Part model, mm, in its own coordinate system. A direction names the side the tool comes from. Give positions to 0.01 mm unless a question says otherwise; leave off trailing zeros. Order: outer loops, then holes, each group sorted by start corner. A loop starts at its lowest first (then second) coordinate and runs counter-clockwise, first axis right, second up. Notation, with made-up numbers: (-2.75, 40) - (44.25, 40) arc R11 ccw to (44.25, 46) - close; hole circle Ø4 at (41.5, -30.5). An arc over 180 degrees is marked (long way). Use one line per item in the form item = value. Start each with the question number.
1. Pin check, flat tips, straight feed: P1, Ø3.5, axis at x = 3, z = 9, coming from the -Y side; P2, Ø1, axis at y = 2, z = 41.5, coming from the +X side. Stop position of each tip, or through.
2. Pull direction Z, two halves, no side cores. Call faces 1 (the face through (-10.24, 1.48, 56.45)), 2 (the face through (61.976, 1, -26)), 3 (the face through (41.406, 1.521, 29.568)): +Z half, -Z half, draft (parallel to the pull), parting line (faces both ways), or undercut.
3. Band-saw the part on C-C, the plane x = 49.5. List the corners of the cut face in (y, z), plus the area to 3 significant figures.
4. Band-saw the part on D-D, the plane y = 1.6. State how many separate pieces and enclosed holes the cut face has, plus the area to 3 significant figures.
5. Tool access for faces 4 (the face through (49.73, 1.48, 17.72)), 5 (the face through (13.631, 1.479, -52.997)): list every direction of +Z, -Z, +X, -X, +Y, -Y with a clear straight run to the whole face (end or side of a thin tool).
6. Drill centre lines: line 1 (X direction, y = 1.25, z = 28.5); line 2 (X direction, y = 0.65, z = -32); line 3 (Z direction, x = -25.5, y = 0.6). Where is each one in solid material? Low to high.
7. Band-saw the part on A-A, the plane x = 9. List the corners of the cut face in (y, z), plus the area to 3 significant figures.
8. Band-saw the part on B-B, the plane z = 15. List the corners of the cut face in (x, y).
from build123d import *
from build123d.topology import SkipClean

# Parameters (mm, degrees)
SKETCH_1_R               = 1.55
SKETCH_1_R_2             = 4
EXTRUDE_1_DEPTH          = 3
EXTRUDE_START            = -3
SKETCH_2_R               = 2.1
EXTRUDE_3_DEPTH          = 3
FILLET_1_R               = 4
FILLET_2_R               = 314
FILLET_3_R               = 314
FILLET_4_R               = 4
CUT_EXTRUDE_2_DEPTH      = 3
EXTRUDE_4_DEPTH          = 3
CUT_EXTRUDE_START        = -10
SKETCH_5_R               = 22.5
CUT_EXTRUDE_3_DEPTH      = 10
SKETCH_6_R               = 13.5
EXTRUDE_5_DEPTH          = 3
EXTRUDE_6_DEPTH          = 3
CUT_EXTRUDE_5_DEPTH      = 98.662684788
CUT_EXTRUDE_5_DEPTH_BACK = 3
SKETCH_9_R               = 1.55
CUT_EXTRUDE_7_DEPTH      = 10
SKETCH_10_W              = 64.519287894
SKETCH_10_H              = 7.041569679
EXTRUDE_7_DEPTH          = 3
SKETCH_11_R              = 1.55
CUT_EXTRUDE_8_DEPTH      = 10


with BuildPart() as part:
    # 草图1 → 凸台-拉伸1 (new body)
    with BuildSketch(Plane(origin=(0, 0, 0), x_dir=(1, 0, 0), z_dir=(0, 1, 0))):
        with BuildLine():
            Line((-27.819418646, 37.14796354), (-55, 11))
            Line((-55, 11), (-55, -11))
            Line((-55, -11), (-27.819418646, -37.14796354))
            ThreePointArc((-27.819418646, -37.14796354), (-23.984664844, -39.630488814), (-19.5, -40.5))
            Line((-19.5, -40.5), (-17.421399483, -40.31860482))
            Line((-17.421399483, -40.31860482), (45.042813224, -34.867481809))
            ThreePointArc((45.042813224, -34.867481809), (58.724014778, -30.74585061), (69.617928959, -21.5))
            Line((69.617928959, -21.5), (19, -21.5))
            ThreePointArc((19, -21.5), (15.464466094, -20.035533906), (14, -16.5))
            Line((14, -16.5), (14, -12.539936204))
            ThreePointArc((14, -12.539936204), (5.5, 0), (14, 12.539936204))
            Line((14, 12.539936204), (14, 16.5))
            ThreePointArc((14, 16.5), (15.464466094, 20.035533906), (19, 21.5))
            Line((19, 21.5), (69.617928959, 21.5))
            ThreePointArc((69.617928959, 21.5), (58.724014778, 30.74585061), (45.042813224, 34.867481809))
            Line((45.042813224, 34.867481809), (-17.421399483, 40.31860482))
            Line((-17.421399483, 40.31860482), (-19.5, 40.5))
            ThreePointArc((-19.5, 40.5), (-23.984664844, 39.630488814), (-27.819418646, 37.14796354))
        make_face()
        with Locations(Location((-29, -28.5, 0), (0, 0, 270))):
            Circle(SKETCH_1_R, mode=Mode.SUBTRACT)
        with Locations(Location((-19.5, -36.5, 0), (0, 0, 270))):
            Circle(SKETCH_1_R, mode=Mode.SUBTRACT)
        with Locations(Location((-19.5, -28.5, 0), (0, 0, 270))):
            Circle(SKETCH_1_R_2, mode=Mode.SUBTRACT)
        with Locations(Location((-10, -28.5, 0), (0, 0, 270))):
            Circle(SKETCH_1_R, mode=Mode.SUBTRACT)
        with Locations(Location((-19.5, -20.5, 0), (0, 0, 270))):
            Circle(SKETCH_1_R, mode=Mode.SUBTRACT)
        with Locations(Location((-46.5, 0, 0), (0, 0, 270))):
            Circle(SKETCH_1_R, mode=Mode.SUBTRACT)
        with Locations(Location((-27.5, 0, 0), (0, 0, 270))):
            Circle(SKETCH_1_R, mode=Mode.SUBTRACT)
        with Locations(Location((0, 0, 0), (0, 0, 270))):
            Circle(SKETCH_1_R, mode=Mode.SUBTRACT)
        with Locations(Location((-29, 28.5, 0), (0, 0, 270))):
            Circle(SKETCH_1_R, mode=Mode.SUBTRACT)
        with Locations(Location((-19.5, 20.5, 0), (0, 0, 270))):
            Circle(SKETCH_1_R, mode=Mode.SUBTRACT)
        with Locations(Location((-19.5, 28.5, 0), (0, 0, 270))):
            Circle(SKETCH_1_R_2, mode=Mode.SUBTRACT)
        with Locations(Location((-10, 28.5, 0), (0, 0, 270))):
            Circle(SKETCH_1_R, mode=Mode.SUBTRACT)
        with Locations(Location((-19.5, 36.5, 0), (0, 0, 270))):
            Circle(SKETCH_1_R, mode=Mode.SUBTRACT)
    extrude(amount=EXTRUDE_1_DEPTH)

    # 草图2 → 凸台-拉伸3 (add)
    with BuildSketch(Plane(origin=(0, 3, 0), x_dir=(1, 0, 0), z_dir=(0, 1, 0)).offset(EXTRUDE_START)):
        with BuildLine():
            Line((-7, 60), (-28.363974347, 36.588878709))
            ThreePointArc((-28.363974347, 36.588878709), (-26.665503977, 38.125775437), (-24.705947863, 39.311942788))
            Line((-24.705947863, 39.311942788), (-19.656872495, 39.177623495))
            Line((-19.656872495, 39.177623495), (-17.421399483, 40.31860482))
            Line((-17.421399483, 40.31860482), (17, 37.314720281))
            Line((17, 37.314720281), (17, 50))
            Line((17, 50), (17, 60))
            Line((17, 60), (-7, 60))
        make_face()
        with Locations(Location((13, 55, 0), (0, 0, 270))):
            Circle(SKETCH_2_R, mode=Mode.SUBTRACT)
        with Locations(Location((-3, 55, 0), (0, 0, 270))):
            Circle(SKETCH_2_R, mode=Mode.SUBTRACT)
    extrude_3 = extrude(amount=EXTRUDE_3_DEPTH)

    # 圆角1
    fillet_1_edges = [part.edges().sort_by_distance(p)[0] for p in [
        (17, 1.5, -37.314720281),
    ]]
    fillet(fillet_1_edges, radius=FILLET_1_R)

    # 圆角2
    # the kernel refuses this fillet: 314 mm, written as the material it adds along each edge
    with BuildSketch(Plane(origin=(-28.100791786, 0, -36.877280051), x_dir=(0.6740732257670936, 0, -0.7386645289330906), z_dir=(0, 1, 0))) as fillet_2_piece_1:
        with BuildLine():
            CenterArc((FILLET_2_R * 0.032536346624, FILLET_2_R), FILLET_2_R, 266.272924122, 3.727075878)
            Line((-FILLET_2_R * 0.0324675326171, FILLET_2_R * 0.0021149887469), (0, 0))
            Line((0, 0), (FILLET_2_R * 0.032536346624, 0))
        make_face()
    extrude(amount=3)

    # 镜向2: 凸台-拉伸3 across plane
    add(extrude_3.mirror(Plane.XY))

    # 圆角3
    # the kernel refuses this fillet: 314 mm, written as the material it adds along each edge
    with BuildSketch(Plane(origin=(-28.100791786, 0, 36.877280051), x_dir=(-0.7206636283184775, 0, -0.6932848871992288), z_dir=(0, 1, 0))) as fillet_3_piece_1:
        with BuildLine():
            CenterArc((FILLET_3_R * 0.0325363466241, FILLET_3_R), FILLET_3_R, 266.272924122, 3.727075878)
            Line((-FILLET_3_R * 0.0324675326171, FILLET_3_R * 0.0021149887469), (0, 0))
            Line((0, 0), (FILLET_3_R * 0.032536346624, 0))
        make_face()
    extrude(amount=3)

    # 圆角4
    fillet_4_edges = [part.edges().sort_by_distance(p)[0] for p in [
        (17, 1.5, 37.314720281),
    ]]
    fillet(fillet_4_edges, radius=FILLET_4_R)

    # 草图3 → 切除-拉伸2 (cut)
    with BuildSketch(Plane.XZ):
        with BuildLine():
            ThreePointArc((-8.686732059, 48.231275591), (-35.637539634, 44.178960889), (-38.911435654, 17.122558906))
            ThreePointArc((-38.911435654, 17.122558906), (-32.411561674, 15.426493388), (-30.715496156, 21.926367368))
            ThreePointArc((-30.715496156, 21.926367368), (-28.823911789, 37.55895518), (-13.252334078, 39.900292563))
            ThreePointArc((-13.252334078, 39.900292563), (-6.804041555, 41.782983067), (-8.686732059, 48.231275591))
        make_face()
    cut_extrude_2 = extrude(amount=-CUT_EXTRUDE_2_DEPTH, mode=Mode.SUBTRACT)

    # 草图4 → 凸台-拉伸4 (add)
    with SkipClean():  # the faces are left unmerged after this step: merging them gives an invalid solid
        with BuildSketch(Plane.XZ):
            with BuildLine():
                Line((-43.624805935, 21.943038922), (-41.535713139, 23.952764967))
                ThreePointArc((-41.535713139, 23.952764967), (-35.617955509, 44.199092655), (-15.534428758, 50.647781937))
                Line((-15.534428758, 50.647781937), (-13.580394358, 52.78905657))
                ThreePointArc((-13.580394358, 52.78905657), (-37.408839455, 45.943436284), (-43.624805935, 21.943038922))
            make_face()
            with BuildLine():
                ThreePointArc((-25.118289886, 40.223259732), (-28.812596517, 37.570586867), (-31.367097826, 33.807729194))
                ThreePointArc((-31.367097826, 33.807729194), (-28.219819959, 36.993214998), (-25.118289886, 40.223259732))
            make_face()
        extrude_4 = extrude(amount=-EXTRUDE_4_DEPTH)

    # 镜向9: 切除-拉伸2, 凸台-拉伸4 across plane
    with SkipClean():  # the faces are left unmerged after this step: merging them gives an invalid solid
        add(cut_extrude_2.mirror(Plane.XY), mode=Mode.SUBTRACT)
        add(extrude_4.mirror(Plane.XY))

    # 草图5 → 切除-拉伸3 (cut)
    with SkipClean():  # the faces are left unmerged after this step: merging them gives an invalid solid
        with BuildSketch(Plane(origin=(0, 3, 0), x_dir=(1, 0, 0), z_dir=(0, 1, 0)).offset(CUT_EXTRUDE_START)):
            with Locations(Location((-19.5, 28.5, 0), (0, 0, 270))):
                Circle(SKETCH_5_R)
            with Locations(Location((-19.5, -28.5, 0), (0, 0, 90))):
                Circle(SKETCH_5_R)
        extrude(amount=CUT_EXTRUDE_3_DEPTH, mode=Mode.SUBTRACT)

    # 草图6 → 凸台-拉伸5 (add)
    with SkipClean():  # the faces are left unmerged after this step: merging them gives an invalid solid
        with BuildSketch(Plane(origin=(0, 3, 0), x_dir=(1, 0, 0), z_dir=(0, 1, 0)).offset(EXTRUDE_START)):
            with BuildLine():
                ThreePointArc((7.831521739, -7.583870604), (77, 0), (7.831521739, 7.583870604))
                ThreePointArc((7.831521739, 7.583870604), (5.5, 0), (7.831521739, -7.583870604))
            make_face()
            with Locations(Location((42, 0, 0), (0, 0, 270))):
                Circle(SKETCH_6_R, mode=Mode.SUBTRACT)
        extrude(amount=EXTRUDE_5_DEPTH)

    # 草图7 → 凸台-拉伸6 (add)
    with SkipClean():  # the faces are left unmerged after this step: merging them gives an invalid solid
        with BuildSketch(Plane(origin=(0, 3, 0), x_dir=(1, 0, 0), z_dir=(0, 1, 0)).offset(EXTRUDE_START)):
            with BuildLine():
                Line((17, 60), (61.975534644, 28.739833258))
                ThreePointArc((61.975534644, 28.739833258), (53.910000161, 32.911273086), (45.042813224, 34.867481809))
                Line((45.042813224, 34.867481809), (20.652249917, 36.995995963))
                ThreePointArc((20.652249917, 36.995995963), (18.051186651, 38.278167206), (17, 40.980851027))
                Line((17, 40.980851027), (17, 60))
            make_face()
            with BuildLine():
                Line((17, -60), (61.975557807, -28.739817159))
                ThreePointArc((61.975557807, -28.739817159), (53.910013423, -32.911268287), (45.042813224, -34.867481809))
                Line((45.042813224, -34.867481809), (20.652249917, -36.995995963))
                ThreePointArc((20.652249917, -36.995995963), (18.051186651, -38.278167206), (17, -40.980851027))
                Line((17, -40.980851027), (17, -60))
            make_face()
        extrude(amount=EXTRUDE_6_DEPTH)

    # 草图8 → 切除-拉伸5 (cut, two sides: drawn at the far end of the back side and taken through both)
    with SkipClean():  # the faces are left unmerged after this step: merging them gives an invalid solid
        with BuildSketch(Plane(origin=(0, 3, 0), x_dir=(1, 0, 0), z_dir=(0, 1, 0)).offset(-CUT_EXTRUDE_5_DEPTH_BACK)):
            with BuildLine():
                Line((61.975534644, 28.739833258), (61.975534644, 22.739833258))
                Line((61.975534644, 22.739833258), (35.963826017, 12.075371781))
                Line((35.963826017, 12.075371781), (35.963826017, -12.075371781))
                Line((35.963826017, -12.075371781), (61.975534644, -22.739833258))
                Line((61.975534644, -22.739833258), (61.975534644, -28.739833258))
                ThreePointArc((61.975534644, -28.739833258), (77, 1.4104e-05), (61.975534644, 28.739833258))
            make_face()
        extrude(amount=CUT_EXTRUDE_5_DEPTH + CUT_EXTRUDE_5_DEPTH_BACK, mode=Mode.SUBTRACT)

    # 草图9 → 切除-拉伸7 (cut)
    with SkipClean():  # the faces are left unmerged after this step: merging them gives an invalid solid
        with BuildSketch(Plane(origin=(0, 3, 0), x_dir=(1, 0, 0), z_dir=(0, 1, 0))):
            with Locations(Location((-53, -9, 0), (0, 0, 270))):
                Circle(SKETCH_9_R)
            with Locations(Location((-53, 9, 0), (0, 0, 270))):
                Circle(SKETCH_9_R)
            with Locations(Location((3, 9, 0), (0, 0, 270))):
                Circle(SKETCH_9_R)
            with Locations(Location((3, -9, 0), (0, 0, 270))):
                Circle(SKETCH_9_R)
        extrude(amount=-CUT_EXTRUDE_7_DEPTH, mode=Mode.SUBTRACT)

    # 草图10 → 凸台-拉伸7 (add)
    with SkipClean():  # the faces are left unmerged after this step: merging them gives an invalid solid
        with BuildSketch(Plane(origin=(0, 3, 0), x_dir=(1, 0, 0), z_dir=(0, 1, 0))):
            with Locations((-17.723905758, 0.445902683)):
                Rectangle(SKETCH_10_W, SKETCH_10_H)
        extrude(amount=-EXTRUDE_7_DEPTH)

    # 草图11 → 切除-拉伸8 (cut)
    with SkipClean():  # the faces are left unmerged after this step: merging them gives an invalid solid
        with BuildSketch(Plane(origin=(0, 3, 0), x_dir=(1, 0, 0), z_dir=(0, 1, 0))):
            with Locations(Location((57.975534644, 25.739833258, 0), (0, 0, 270))):
                Circle(SKETCH_11_R)
            with Locations(Location((42, 31, 0), (0, 0, 270))):
                Circle(SKETCH_11_R)
            with Locations(Location((9, 15, 0), (0, 0, 270))):
                Circle(SKETCH_11_R)
        cut_extrude_8 = extrude(amount=-CUT_EXTRUDE_8_DEPTH, mode=Mode.SUBTRACT)

    # 镜向10: 切除-拉伸8 across plane
    with SkipClean():  # the faces are left unmerged after this step: merging them gives an invalid solid
        add(cut_extrude_8.mirror(Plane.XY), mode=Mode.SUBTRACT)


solid = part.part
From the geometry:
q1.P1 = 0
q1.P2 = 44.34
q2.face_1 = +Z half
q2.face_2 = draft
q2.face_3 = undercut
q3.outline = (0, -37.41) - (3, -37.41) - (3, -17.63) - (0, -17.63) - close; (0, 17.63) - (3, 17.63) - (3, 37.41) - (0, 37.41) - close
q3.area = 119 mm²
q4.separate_pieces = 1
q4.enclosed_holes = 16
q4.area = 6,640 mm²
q5.face_4 = +X, +Y, -Y
q5.face_5 = +Y, -Y
q6.line_1 = -44.5 to -42, 3 to 61.98
q6.line_2 = -44.25 to -41.73, 2.73 to 40.82, 43.18 to 57.28
q6.line_3 = -52.77 to -50.19, -6.81 to 6.81, 50.19 to 52.77
q7.outline = (0, -60) - (3, -60) - (3, -16.55) - (0, -16.55) - close; (0, -13.45) - (3, -13.45) - (3, 13.45) - (0, 13.45) - close; (0, 16.55) - (3, 16.55) - (3, 60) - (0, 60) - close
q7.area = 341 mm²
q8.outline = (-50.84, 0) - (-37.5, 0) - (-37.5, 3) - (-50.84, 3) - close; (-1.5, 0) - (7.45, 0) - (7.45, 3) - (-1.5, 3) - close; (10.55, 0) - (43.1, 0) - (43.1, 3) - (10.55, 3) - close
